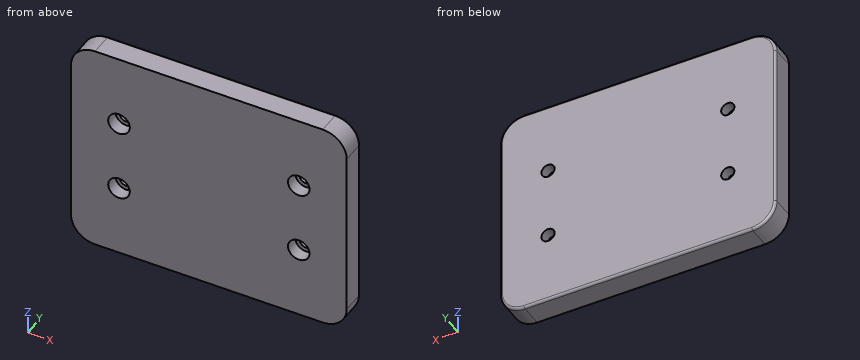
Autodesk Inventor part; units mm, degrees
ref_plane "YZ Plane" through (0, 0, 0) normal (1, 0, 0) x (0, 1, 0)
ref_plane "XZ Plane" through (0, 0, 0) normal (0, 1, 0) x (-1, 0, 0)
ref_plane "XY Plane" through (0, 0, 0) normal (0, 0, 1) x (1, 0, 0)
sketch "Sketch1" plane through (0, 0, 0) normal (0, 1, 0) x (-1, 0, 0)
  line L0 (115, 90) -> (-115, 90)
  line L1 (-115, 90) -> (-115, -90)
  line L2 (-115, -90) -> (115, -90)
  line L3 (115, -90) -> (115, 90)
  line L4 (115, 90) -> (-115, -90) construction
  line L5 (-115, 90) -> (115, -90) construction
  point P0 (0, 0)
  dimension "d0" = 230
  dimension "d1" = 180
extrude "Extrusion1" add sketch "Sketch1" along normal blind 20
fillet "Fillet1" radius 2 4 edges at (0, 20, 90) (115, 20, 0) (0, 20, -90) (-115, 20, 0)
fillet "Fillet2" radius 20 8 edges at (-114.4142, 19.4142, 89.4142) (-115, 9, 90) (114.4142, 19.4142, 89.4142) (115, 9, 90) (-115, 9, -90) (-114.4142, 19.4142, -89.4142) (114.4142, 19.4142, -89.4142) (115, 9, -90)
sketch "Sketch2" plane through (0, 20, 0) normal (0, 1, 0) x (1, 0, 0)
  line L0 (75, 30) -> (0, 0)
  circle A0 centre (75, 30) radius 5.5
  dimension "d6" = 11
extrude "Extrusion2" cut sketch "Sketch2" against normal blind 20
sketch "Sketch3" plane through (0, 0, 0) normal (0, -1, 0) x (1, 0, 0)
  circle A0 centre (75, -30) radius 5.5
  circle A1 centre (75, -30) radius 9
  point P0 (0, 0)
  dimension "d9" = 18
extrude "Extrusion3" cut sketch "Sketch3" against normal blind 11 contours A0 | A1
mirror "Mirror1" about plane through (0, 0, 0) normal (0, 0, 1) of "Extrusion2", "Extrusion3"
mirror "Mirror2" about plane through (0, 0, 0) normal (1, 0, 0) of "Extrusion2", "Extrusion3", "Mirror1"
properties part number "stand" material "Wood (Birch)"
Read the model definition and answer for the solid it produces. Units are mm, in the model's axes. Round coordinates to 2 decimals unless told otherwise and drop trailing zeros. Order: outer loops, then holes, each group sorted by start corner. A loop starts at its lowest first (then second) coordinate and runs counter-clockwise, first axis right, second up. Notation, with made-up numbers: (-33, 41.5) - (-23, 41.5) arc R12 cw to (-23, 54.5) - close; hole circle Ø3 at (38, 4). An arc over 180 degrees is marked (long way). Use one line per item in the form item = value. Start each with the question number.
(1) The part is cut by section A-A (z = 30). Give the vertices of the cut face in (x, y).
(2) The part is cut by section B-B (x = 75). Give the vertices of the cut face in (y, z), then the cut area to 3 significant figures.
(3) Find the intervals of material crossed by line 1 along Z through (x, y) = (-75, 15.25); line 2 along Z through (x, y) = (-75, 8.5); line 3 along X through (y, z) = (13.5, -34), in increasing order. Write a range as from..to.
(4) Flat-ended cylindrical pins translate along their axes: pin 1 Ø20.5 at (x, z) = (-75, 30) entering from +Y; pin 2 Ø14.5 at (x, z) = (75, 30) entering from -Y. Find the tip coordinate at first contact, or state that the pin passes through.
Checked values:
q1.outline = (-115, 0) - (-84, 0) - (-84, 11) - (-80.5, 11) - (-80.5, 20) - (-113, 20) arc R2 ccw to (-115, 18) - close; (-69.5, 11) - (-66, 11) - (-66, 0) - (66, 0) - (66, 11) - (69.5, 11) - (69.5, 20) - (-69.5, 20) - close; (80.5, 11) - (84, 11) - (84, 0) - (115, 0) - (115, 18) arc R2 ccw to (113, 20) - (80.5, 20) - close
q2.outline = (0, -90) - (18, -90) arc R2 ccw to (20, -88) - (20, -35.5) - (11, -35.5) - (11, -39) - (0, -39) - close; (0, -21) - (11, -21) - (11, -24.5) - (20, -24.5) - (20, 24.5) - (11, 24.5) - (11, 21) - (0, 21) - close; (0, 39) - (11, 39) - (11, 35.5) - (20, 35.5) - (20, 88) arc R2 ccw to (18, 90) - (0, 90) - close
q2.area = 3,000 mm^2
q3.line_1 = -90..-35.5, -24.5..24.5, 35.5..90
q3.line_2 = -90..-39, -21..21, 39..90
q3.line_3 = -115..-78.77, -71.23..71.23, 78.77..115
q4.pin_1 = 20
q4.pin_2 = 11
